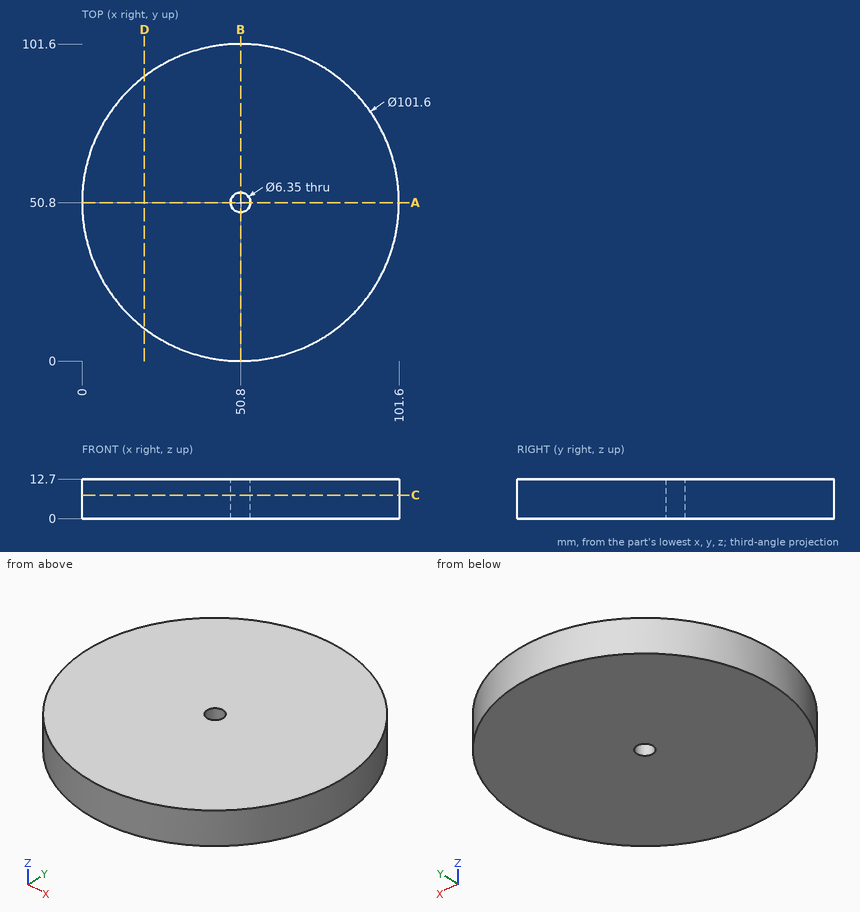
Source: three-view drawing plus pictorial views. Frame: mm from the lowest corner of the part. Coordinates: 2 decimals unless noted, no trailing zeros. Loops run counter-clockwise (first coordinate to the right, second up) from the corner with the lowest first, then second, coordinate; pieces in that order, holes last. Notation, with made-up numbers: (-1.5, 81) - (54.5, 81) arc R8 cw to (54.5, 96) - close; hole circle Ø5 at (61, 37.5). An arc over 180 degrees is marked (long way). One line per item, written item: value. Start each with the question number.
1. Contact query for flat-ended pins moving along their axis: P1, Ø2, axis at y = 49, z = 2.5, coming from the +X side; P2, Ø1.5, axis at x = 17, z = 2.5, coming from the +Y side; P3, Ø1, axis at y = 16.5, z = 4.5, coming from the +X side. Output: stop coordinate, or through.
2. Section A-A (y = 50.8). Return the cut outline in (x, z) (3 decimals).
3. Section C-C (z = 7.5). Return the cut outline in (x, y) (3 decimals).
4. Section D-D (x = 20). Return the cut outline in (y, z).
5. Ray query, L1, parallel to Y at x = 50.8, z = 6.25 (3 decimals); L2, parallel to X at y = 37, z = 5.25; L3, parallel to X at y = 64, z = 2.25. Return the intervals inside material, ascending.
Verdict:
1. P1: stops at x = 101.59
1. P2: stops at y = 89.38
1. P3: stops at x = 88.72
2. outline: (0, 0) - (47.625, 0) - (47.625, 12.7) - (0, 12.7) - close; (53.975, 0) - (101.6, 0) - (101.6, 12.7) - (53.975, 12.7) - close
3. outline: circle Ø101.6 at (50.8, 50.8); hole circle Ø6.35 at (50.8, 50.8)
4. outline: (10.4, 0) - (91.2, 0) - (91.2, 12.7) - (10.4, 12.7) - close
5. L1: y = 0 to 47.625, 53.975 to 101.6
5. L2: x = 1.91 to 99.69
5. L3: x = 1.74 to 99.86
